Here's the drawing with two shaded views (mm, measured from the low corner). I have some questions. Round coordinates to 2 decimals unless told otherwise and drop trailing zeros. Write each loop counter-clockwise with the first axis right and the second up, starting at its lowest first coordinate (ties: lowest second). Pieces come first, ordered by that corner, then holes. Notation, with made-up numbers: (84.25, -14.5) - (117.25, -14.5) arc R26 cw to (117.25, 18.5) - close; hole circle Ø10 at (49.5, 50.25). An arc over 180 degrees is marked (long way). Return JSON: item names as keys, results as strings. Group by question number.
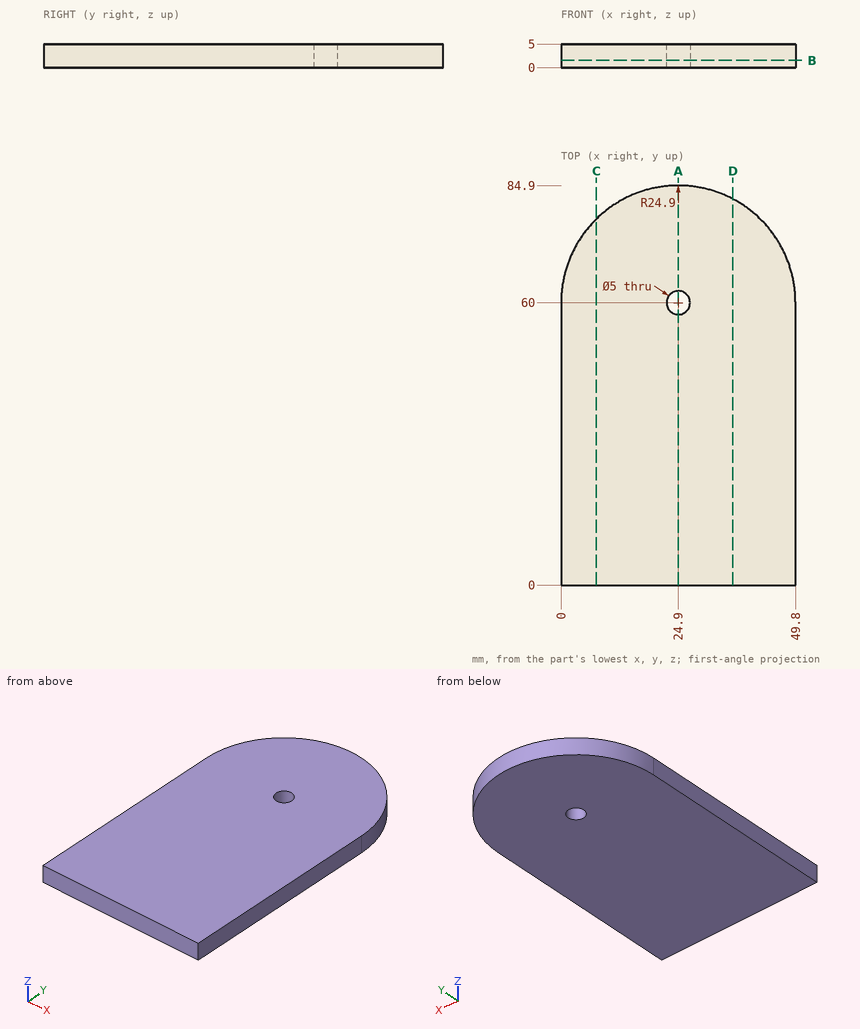
1) Will this pin go through, and if not, where does the flat tip stop? pin 1 Ø2 at (y, z) = (62.5, 4) entering from -X.
2) Imagine slicing it at B-B (z = 1.5). Please give me the cut outline in (x, y), plus the area to 3 significant figures.
3) Imagine slicing it at A-A (x = 24.9). Please give me the cut outline in (y, z).
4) Imagine slicing it at D-D (x = 36.5). Please give me the cut outline in (y, z).
5) Imagine slicing it at C-C (x = 7.5). Please give me the cut outline in (y, z), plus the area to 3 significant figures.
6) I need wall thicknesses on line 1 along Y through (x, z) = (24.9, 1.65); line 2 along Y through (x, z) = (14, 1.05); line 3 along X through (y, z) = (61, 2.7). Which ranges of each line are inside material? Lowest first, please.
Results found:
{
 "1": {"pin 1": "stops at x = 0.05"},
 "2": {"outline": "(0, 0) - (49.8, 0) - (49.8, 60) arc R24.9 ccw to (0, 60) - close; hole circle Ø5 at (24.9, 60)", "area": "3,940 mm²"},
 "3": {"outline": "(0, 0) - (57.5, 0) - (57.5, 5) - (0, 5) - close; (62.5, 0) - (84.9, 0) - (84.9, 5) - (62.5, 5) - close"},
 "4": {"outline": "(0, 0) - (82.03, 0) - (82.03, 5) - (0, 5) - close"},
 "5": {"outline": "(0, 0) - (77.81, 0) - (77.81, 5) - (0, 5) - close", "area": "389 mm²"},
 "6": {"line 1": "y = 0 to 57.5, 62.5 to 84.9", "line 2": "y = 0 to 82.39", "line 3": "x = 0.02 to 22.61, 27.19 to 49.78"}
}
